Could you check a few things on this model? Use its own coordinates, in mm. Round coordinates to 2 decimals unless told otherwise and drop trailing zeros. Loops run counter-clockwise (first coordinate to the right, second up) from the corner with the lowest first, then second, coordinate; pieces in that order, holes last. Notation, with made-up numbers: (-13, 54) -> (13, 54) arc R21 cw to (13, 60) -> close; hole circle Ø8 at (43.5, -33). An arc over 180 degrees is marked (long way). Put each result on its own line as item: value. Start each with the question number.
1. Imagine slicing it at C-C, the plane z = 0. Count the separate pieces of the cut face and the enclosed holes in it, and give its area (3 significant figures).
2. I'm going to push flat-ended pins straight in: P1, Ø13.5, axis at y = -1121.5, z = 0, coming from the +X side; P2, Ø12, axis at x = -12, z = 15, coming from the +Y side. Where does each tip first touch, or does it pass through?
3. Imagine slicing it at B-B, the plane x = 15. Please give me the cut outline in (y, z).
4. I need wall thicknesses on line 1 (Z direction, x = -4.5, y = -382); line 2 (Z direction, x = 23.7, y = -316.5). Which ranges of each line are inside material? Lowest first, please. Write a range as [from, to].
5. Imagine slicing it at A-A, the plane y = -174.5. Please give me the cut outline in (x, z).
Autodesk Inventor part; units mm, degrees
ref_plane "YZ Plane" through (0, 0, 0) normal (1, 0, 0) x (0, 1, 0)
ref_plane "XZ Plane" through (0, 0, 0) normal (0, 1, 0) x (-1, 0, 0)
ref_plane "XY Plane" through (0, 0, 0) normal (0, 0, 1) x (1, 0, 0)
sketch "Sketch9" plane through (0, 0, 0) normal (0, 1, 0) x (-1, 0, 0)
  line L0 (25, 25) -> (-25, 25)
  line L1 (-25, 25) -> (-25, -25)
  line L2 (-25, -25) -> (25, -25)
  line L3 (25, -25) -> (25, 25)
  line L4 (25, 25) -> (-25, -25) construction
  line L5 (-25, 25) -> (25, -25) construction
  line L6 (-23, 23) -> (23, 23)
  line L7 (23, 23) -> (23, -23)
  line L8 (23, -23) -> (-23, -23)
  line L9 (-23, -23) -> (-23, 23)
  point P0 (0, 0)
  dimension "d172" = 50
  dimension "d173" = 50
  dimension "d174" = 2
extrude "Extrusion3" add sketch "Sketch9" against normal blind 1365
sketch "Sketch10" plane through (0, 0, 0) normal (1, 0, 0) x (0, 1, 0)
  line L0 (0, 25) -> (0, -25) construction
  line L1 (0, 25) -> (-1365, 25) construction
  line L2 (-1365, -25) -> (-1365, 25) construction
  line L3 (0, -25) -> (-1365, -25) construction
  line L4 (-1360, 8.5) -> (-1343, 8.5)
  line L5 (-1343, 8.5) -> (-1343, -8.5)
  line L6 (-1343, -8.5) -> (-1360, -8.5)
  line L7 (-1360, -8.5) -> (-1360, 8.5)
  line L8 (-1360, 8.5) -> (-1343, -8.5) construction
  line L9 (-1343, 8.5) -> (-1360, -8.5) construction
  circle A0 centre (-1351.5, 0) radius 8.5
  line L10 (0, 25) -> (0, -25)
  point P0 (0, 0)
  point P1 (0, 0)
  point P2 (-1365, 0)
  dimension "d177" = 17
  dimension "d178" = 17
  dimension "d191" = 5
extrude "Extrusion4" cut sketch "Sketch10" along normal through all contours A0
pattern_linear "Rectangular Pattern4" count 12 spacing 115 along (0, 1, 0) of "Extrusion4"
properties part number "TKS 3531 FDS WAY tube1" material "Stainless Steel"
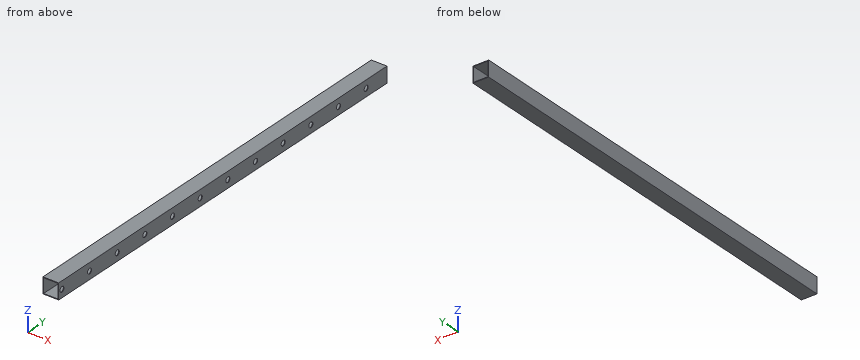
Entries:
1. separate pieces: 14
1. enclosed holes: 0
1. area: 5,050 mm^2
2. P1: x = -23
2. P2: through
3. outline: (-1365, -25) -> (0, -25) -> (0, -23) -> (-1365, -23) -> close; (-1365, 23) -> (0, 23) -> (0, 25) -> (-1365, 25) -> close
4. line 1: [-25, -23], [23, 25]
4. line 2: [-25, -8.5], [8.5, 25]
5. outline: (-25, -25) -> (25, -25) -> (25, 25) -> (-25, 25) -> close; hole (-23, -23) -> (23, -23) -> (23, 23) -> (-23, 23) -> close
